CAD build for the part. Positions are in the model's coordinates, mm. A direction names the side the tool comes from. Round coordinates to 2 decimals unless told otherwise and drop trailing zeros. Loops run counter-clockwise (first coordinate to the right, second up) from the corner with the lowest first, then second, coordinate; pieces in that order, holes last.
```python
from build123d import *

# Parameters (mm, degrees)
SKETCH_1_R      = 1.05
EXTRUDE_1_DEPTH = 0.9


with BuildPart() as part:
    # Эскиз1 → Бобышка-Вытянуть1 (new body)
    with BuildSketch(Plane.XY):
        with BuildLine():
            ThreePointArc((-6.982577353, 2.73744653), (-7.5, 0), (-6.982577353, -2.73744653))
            Line((-6.982577353, -2.73744653), (-8.765394532, -5.28357333))
            ThreePointArc((-8.765394532, -5.28357333), (-8.485281374, -8.485281374), (-5.28357333, -8.765394532))
            Line((-5.28357333, -8.765394532), (-2.73744653, -6.982577353))
            ThreePointArc((-2.73744653, -6.982577353), (0, -7.5), (2.73744653, -6.982577353))
            Line((2.73744653, -6.982577353), (5.28357333, -8.765394532))
            ThreePointArc((5.28357333, -8.765394532), (8.485281374, -8.485281374), (8.765394532, -5.28357333))
            Line((8.765394532, -5.28357333), (6.982577353, -2.73744653))
            ThreePointArc((6.982577353, -2.73744653), (7.5, 0), (6.982577353, 2.73744653))
            Line((6.982577353, 2.73744653), (8.765394532, 5.28357333))
            ThreePointArc((8.765394532, 5.28357333), (8.485281374, 8.485281374), (5.28357333, 8.765394532))
            Line((5.28357333, 8.765394532), (2.73744653, 6.982577353))
            ThreePointArc((2.73744653, 6.982577353), (0, 7.5), (-2.73744653, 6.982577353))
            Line((-2.73744653, 6.982577353), (-5.28357333, 8.765394532))
            ThreePointArc((-5.28357333, 8.765394532), (-8.485281374, 8.485281374), (-8.765394532, 5.28357333))
            Line((-8.765394532, 5.28357333), (-6.982577353, 2.73744653))
        make_face()
        with Locations((-6.717514421, -6.717514421)):
            Circle(SKETCH_1_R, mode=Mode.SUBTRACT)
        with Locations((6.717514421, -6.717514421)):
            Circle(SKETCH_1_R, mode=Mode.SUBTRACT)
        with Locations((-6.717514421, 6.717514421)):
            Circle(SKETCH_1_R, mode=Mode.SUBTRACT)
        with Locations((6.717514421, 6.717514421)):
            Circle(SKETCH_1_R, mode=Mode.SUBTRACT)
    extrude(amount=EXTRUDE_1_DEPTH)


solid = part.part
```
Item 1: Cut at C-C, the plane y = 8.25. Give the cut face in (x, z).
Answers follow:
outline: (-8.69, 0) - (-4.55, 0) - (-4.55, 0.9) - (-8.69, 0.9) - close; (4.55, 0) - (8.69, 0) - (8.69, 0.9) - (4.55, 0.9) - close
Item 2: Cut at A-A, the plane x = 6. Give the cut face in (y, z), plus the area to 3 significant figures.
Answers follow:
outline: (-9.11, 0) - (-7.48, 0) - (-7.48, 0.9) - (-9.11, 0.9) - close; (-5.95, 0) - (5.95, 0) - (5.95, 0.9) - (-5.95, 0.9) - close; (7.48, 0) - (9.11, 0) - (9.11, 0.9) - (7.48, 0.9) - close
area: 13.6 mm2
Item 3: Cut at D-D, the plane y = 0. Give the cut face in (x, z).
Answers follow:
outline: (-7.5, 0) - (7.5, 0) - (7.5, 0.9) - (-7.5, 0.9) - close
Item 4: Cut at B-B, the plane z = 0.65. Give the cut face in (x, y), plus the area to 3 significant figures.
Answers follow:
outline: (-8.77, -5.28) arc R2.5 ccw to (-5.28, -8.77) - (-2.74, -6.98) arc R7.5 ccw to (2.74, -6.98) - (5.28, -8.77) arc R2.5 ccw to (8.77, -5.28) - (6.98, -2.74) arc R7.5 ccw to (6.98, 2.74) - (8.77, 5.28) arc R2.5 ccw to (5.28, 8.77) - (2.74, 6.98) arc R7.5 ccw to (-2.74, 6.98) - (-5.28, 8.77) arc R2.5 ccw to (-8.77, 5.28) - (-6.98, 2.74) arc R7.5 ccw to (-6.98, -2.74) - close; hole circle Ø2.1 at (-6.72, -6.72); hole circle Ø2.1 at (-6.72, 6.72); hole circle Ø2.1 at (6.72, -6.72); hole circle Ø2.1 at (6.72, 6.72)
area: 250 mm2
Item 5: Two-plate mould, pull along X, no slides. Class faces 4 (the cylindrical face through (7.5, 0, 0.4)), 5 (the flat face through (-7.89, 4.03, 0.44)), 6 (the flat face through (4.03, 7.89, 0.44)): released by +X, released by -X, zero draft, split by the parting line, or undercut.
Answers follow:
face 4: released by +X
face 5: released by -X
face 6: undercut
Item 6: Probe line 1 (Y direction, x = -6.75, z = 0.8); line 2 (X direction, y = 6, z = 0.85). List the from-to ranges inside material, lowest first.
Answers follow:
line 1: y = -9.22 to -7.77, -5.67 to 5.67, 7.77 to 9.22
line 2: x = -9.11 to -7.48, -5.95 to 5.95, 7.48 to 9.11
Item 7: 3-axis set-ups, long thin cutter, end or side, ignore diameter. For faces 1 (the flat face through (-3.99, 7.86, 0.44)), 2 (the flat face through (7.89, -4.03, 0.44)), 3 (the flat face through (-4.03, -7.89, 0.44)): which of +Z, -Z, +X, -X, +Y, -Y reach the whole face in a straight line?
Answers follow:
face 1: +Z, -Z, +Y
face 2: +Z, -Z, +X
face 3: +Z, -Z, -Y
